Work out the finished part from the listing and answer in its coordinate system (mm). A direction names the side the tool comes from. Round coordinates to 2 decimals unless told otherwise and drop trailing zeros. Order: outer loops, then holes, each group sorted by start corner. A loop starts at its lowest first (then second) coordinate and runs counter-clockwise, first axis right, second up. Notation, with made-up numbers: (45.25, 6) -> (85.25, 6) arc R24 ccw to (85.25, 36) -> close; hole circle Ø3 at (38.25, -4.75). An arc over 180 degrees is marked (long way). Use a Markdown table: item, result. Add a question column.
Item 1: A cutting plane is placed at C-C, the plane z = -1.5. Determine the outline of the cut face in (x, y).
Item 2: Flat-ended cylindrical pins translate along their axes: P1, Ø6, axis at x = -19, z = 10, coming from the +Y side; P2, Ø5.5, axis at x = -22.86, y = -13.2, coming from the -Z side; P3, Ø4, axis at x = 2, z = -11.5, coming from the -Y side. Find the tip coordinate at first contact, or state that the pin passes through.
Item 3: Find the intervals of material crossed by L1, parallel to Y at x = 0, z = 18; L2, parallel to Y at x = 0, z = 9; L3, parallel to Z at x = -24.5, y = 3.5, in increasing order. Write a range as [from, to].
Item 4: A cutting plane is placed at B-B, the plane y = 0. Determine the outline of the cut face in (x, z).
Item 5: A tool of negligible diameter and unlimited length cuts with its end or side. For faces 1 (the cylindrical face through (-0.09, 24.3, 17.04)), 2 (the flat face through (21, -7, 14)), from which of +Z, -Z, +X, -X, +Y, -Y can it reach the whole face along a straight path? Write none if from no direction.
Item 6: A cutting plane is placed at D-D, the plane z = 15.5. Determine the outline of the cut face in (x, y).
Item 7: For a pull along X with two mould halves and no side action, classify faces 3 (the cylindrical face through (-24.28, -14.75, 17.04)), 4 (the cylindrical face through (-4.336, -19.524, -3.269)), 5 (the flat face through (6, -18, -20)) as +X half, -X half, draft (parallel to the pull), parting line (faces both ways), or undercut.
Item 8: A cutting plane is placed at A-A, the plane x = 0. Determine the outline of the cut face in (y, z), plus the area to 3 significant figures.
from build123d import *

# Parameters (mm, degrees)
SKETCH1_R           = 20
SKETCH1_R_2         = 17.5
BOSS_EXTRUDE1_DEPTH = 20
SKETCH2_R           = 32
SKETCH2_R_2         = 20
BOSS_EXTRUDE2_DEPTH = 6
SKETCH4_W           = 2.1
SKETCH4_H           = 6
CIRPATTERN1_COUNT   = 3
CHAMFER1_SIZE       = 1
FILLET3_R           = 1


with BuildPart() as part:
    # Sketch1 → Boss-Extrude1 (new body, symmetric)
    with BuildSketch(Plane.XY):
        Circle(SKETCH1_R)
        Circle(SKETCH1_R_2, mode=Mode.SUBTRACT)
    extrude(amount=BOSS_EXTRUDE1_DEPTH, both=True)

    # Chamfer1
    chamfer1_edges = [part.edges().sort_by_distance(p)[0] for p in [
        (-17.5, 0, -20),
    ]]
    chamfer(chamfer1_edges, length=CHAMFER1_SIZE)


with BuildPart() as body_2:
    # Sketch2 → Boss-Extrude2 (new body)
    with BuildSketch(Plane.XY.offset(20)):
        Circle(SKETCH2_R)
        Circle(SKETCH2_R_2, mode=Mode.SUBTRACT)
    extrude(amount=-BOSS_EXTRUDE2_DEPTH)

    # Sketch4 → M5 Tapped Hole1 (revolve, cut)
    with BuildSketch(Plane(origin=(0, 26.4, 14), x_dir=(0, 1, 0), z_dir=(1, 0, 0))):
        with Locations((1.05, 3)):
            Rectangle(SKETCH4_W, SKETCH4_H)
    m5_tapped_hole1 = revolve(axis=Axis((0, 26.4, 7.65), (0, 0, 1)), mode=Mode.SUBTRACT)

    # CirPattern1: M5 Tapped Hole1 ×3 about axis
    cirpattern1_axis = Axis((0, 0, 0), (0, 0, 1))
    for i in range(1, CIRPATTERN1_COUNT):
        add(m5_tapped_hole1.rotate(cirpattern1_axis, i * 360 / CIRPATTERN1_COUNT), mode=Mode.SUBTRACT)


with BuildPart() as part_1:
    add(part.part)

    # Combine1: union body 2
    add(body_2.part)

    # Fillet3
    fillet3_edges = [part_1.edges().sort_by_distance(p)[0] for p in [
        (-20, 0, 14),
    ]]
    fillet(fillet3_edges, radius=FILLET3_R)


solid = part_1.part
Reported:
| question | item | result |
|---|---|---|
| 1 | outline | circle Ø40 at (0, 0); hole circle Ø35 at (0, 0) |
| 2 | P1 | y = 12 |
| 2 | P2 | z = 14 |
| 2 | P3 | y = -20 |
| 3 | L1 | [-32, -17.5], [17.5, 24.3], [28.5, 32] |
| 3 | L2 | [-20, -17.5], [17.5, 20] |
| 3 | L3 | [14, 20] |
| 4 | outline | (-32, 14) -> (-21, 14) arc R1 cw to (-20, 13) -> (-20, -20) -> (-18.5, -20) -> (-17.5, -19) -> (-17.5, 20) -> (-32, 20) -> close; (17.5, -19) -> (18.5, -20) -> (20, -20) -> (20, 13) arc R1 cw to (21, 14) -> (32, 14) -> (32, 20) -> (17.5, 20) -> close |
| 5 | face 1 | +Z, -Z |
| 5 | face 2 | -Z |
| 6 | outline | circle Ø64 at (0, 0); hole circle Ø4.2 at (-22.86, -13.2); hole circle Ø35 at (0, 0); hole circle Ø4.2 at (0, 26.4); hole circle Ø4.2 at (22.86, -13.2) |
| 7 | face 3 | undercut |
| 7 | face 4 | parting line |
| 7 | face 5 | draft |
| 8 | outline | (-32, 14) -> (-21, 14) arc R1 cw to (-20, 13) -> (-20, -20) -> (-18.5, -20) -> (-17.5, -19) -> (-17.5, 20) -> (-32, 20) -> close; (17.5, -19) -> (18.5, -20) -> (20, -20) -> (20, 13) arc R1 cw to (21, 14) -> (24.3, 14) -> (24.3, 20) -> (17.5, 20) -> close; (28.5, 14) -> (32, 14) -> (32, 20) -> (28.5, 20) -> close |
| 8 | area | 318 mm² |
